Study the drawing (mm; zero at the part's minimum x, y, z) and answer. Give positions to 0.01 mm unless a question says otherwise; leave off trailing zeros. Order: outer loops, then holes, each group sorted by start corner. A loop starts at its lowest first (then second) coordinate and runs counter-clockwise, first axis right, second up.
Item 1: A cutting plane is placed at B-B (y = 6). Write down the section's boundary in (x, z), plus the area to 3 significant figures.
Item 2: A cutting plane is placed at A-A (x = 4.5). Write down the section's boundary in (y, z).
Item 3: Find the intervals of material crossed by line 1 along Y through (x, z) = (0.75, 7.5); line 2 along Z through (x, y) = (2.5, 16.25); line 3 along Y through (x, z) = (6, 17), in increasing order.
Item 4: The mould has two halves that part along Z. Classify the marked faces 1, 2 and 3: +Z half, -Z half, draft (parallel to the pull), parting line (faces both ways), or undercut.
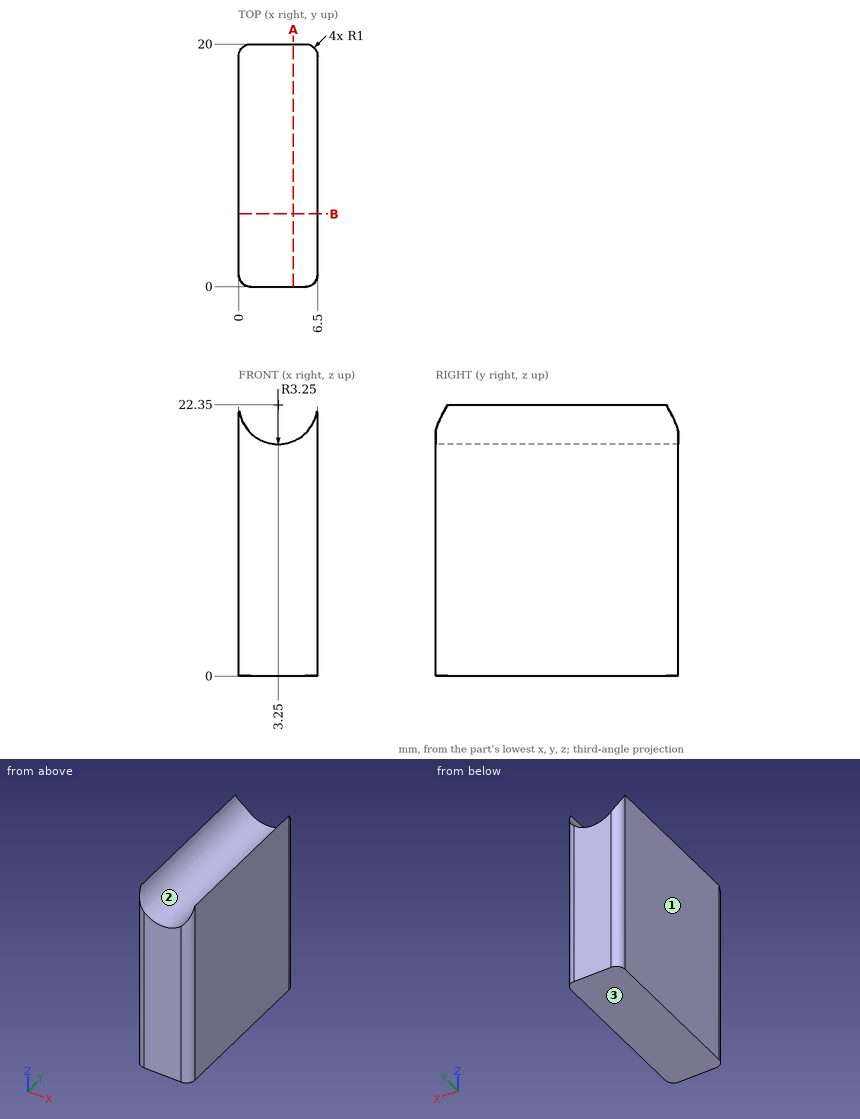
Response values:
1. outline: (0, 0) - (6.5, 0) - (6.5, 22.35) arc R3.25 cw to (0, 22.35) - close
1. area: 129 mm2
2. outline: (0, 0) - (20, 0) - (20, 19.35) - (0, 19.35) - close
3. line 1: y = 0.03 to 19.97
3. line 2: z = 0 to 19.19
3. line 3: y = 0.13 to 19.87
4. face 1: draft
4. face 2: +Z half
4. face 3: -Z half
